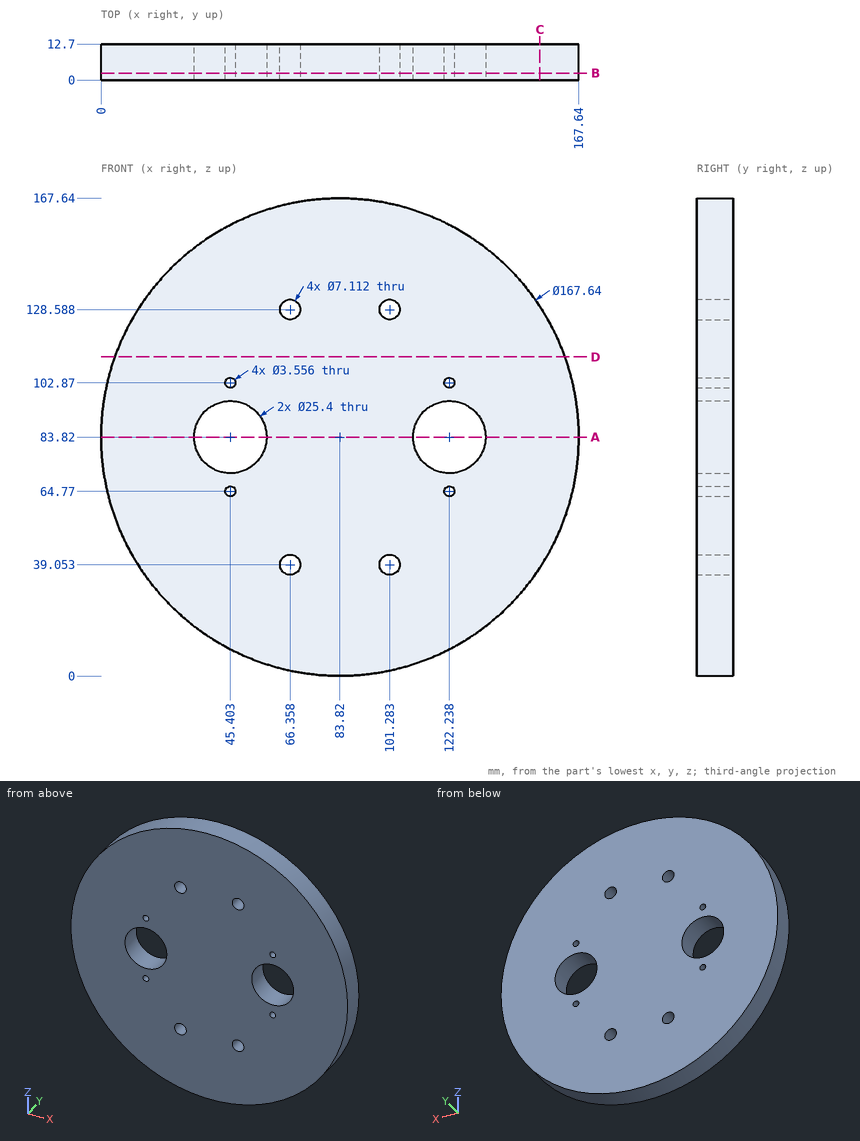
Check sheet for the drawn part. Datum: minimum x, y, z corner. Units: mm. Coordinates: 2 decimals unless noted, no trailing zeros. Loops run counter-clockwise (first coordinate to the right, second up) from the corner with the lowest first, then second, coordinate; pieces in that order, holes last. Notation, with made-up numbers: (7.25, 21.5) -> (37.25, 21.5) arc R20 cw to (37.25, 42.5) -> close; hole circle Ø4 at (13, -9.75). An arc over 180 degrees is marked (long way). Answer in a Markdown table with one row per item.
1. Go/stop test with flat-tipped pins: pin 1 (2 mm diameter, centred on y = 7.5, z = 52.5, fed in from -X) (1 decimal); pin 2 (1 mm diameter, centred on y = 1.5, z = 145.5, fed in from -X) (1 decimal); pin 3 (4 mm diameter, centred on y = 8.5, z = 91.5, fed in from +X). Record where each tip stops, or that it passes through.
Check values:
| item | result |
|---|---|
| pin 1 | stops at x = 5.7 |
| pin 2 | stops at x = 26.5 |
| pin 3 | stops at x = 167.45 |
2. Sectioned sample at B-B, the plane y = 2.5. Give the number of separate pieces and of enclosed holes in the cut face, then the cut area to 3 significant figures.
Check values:
| item | result |
|---|---|
| separate pieces | 1 |
| enclosed holes | 10 |
| area | 20,900 mm2 |
3. Sectioned sample at D-D, the plane z = 112. Record the boundary of the cut face in (x, y), then the cut area to 4 significant figures.
Check values:
| item | result |
|---|---|
| outline | (4.88, 0) -> (162.76, 0) -> (162.76, 12.7) -> (4.88, 12.7) -> close |
| area | 2,005 mm2 |
4. Sectioned sample at C-C, the plane x = 154. Record the boundary of the cut face in (y, z).
Check values:
| item | result |
|---|---|
| outline | (0, 37.99) -> (12.7, 37.99) -> (12.7, 129.65) -> (0, 129.65) -> close |
5. Material ranges on line 1 along Z through (x, y) = (100, 9) (1 decimal); line 2 along Z through (x, y) = (118, 8.25) (1 decimal); line 3 along Z through (x, y) = (51.5, 10.75), recorded low to high. Write a range as [from, to].
Check values:
| item | result |
|---|---|
| line 1 | z = [1.6, 35.7], [42.4, 125.3], [131.9, 166.1] |
| line 2 | z = [7.3, 71.8], [95.8, 160.4] |
| line 3 | z = [6.48, 72.68], [94.96, 161.16] |
6. Sectioned sample at A-A, the plane z = 83.82. Record the boundary of the cut face in (x, y).
Check values:
| item | result |
|---|---|
| outline | (0, 0) -> (32.7, 0) -> (32.7, 12.7) -> (0, 12.7) -> close; (58.1, 0) -> (109.54, 0) -> (109.54, 12.7) -> (58.1, 12.7) -> close; (134.94, 0) -> (167.64, 0) -> (167.64, 12.7) -> (134.94, 12.7) -> close |
